Geometry check sheet. Reference: drawing and pictorial views, mm from the part's lowest x, y, z. A direction names the side the tool comes from. Give positions to 0.01 mm unless a question says otherwise; leave off trailing zeros. Write each loop counter-clockwise with the first axis right and the second up, starting at its lowest first coordinate (ties: lowest second). Pieces come first, ordered by that corner, then holes. Notation, with made-up numbers: (84, 12.5) -> (113, 12.5) arc R25 ccw to (113, 31.5) -> close; hole circle Ø9 at (2.5, 57.25). An arc over 180 degrees is marked (long way). Answer as CSV lines item,"result".
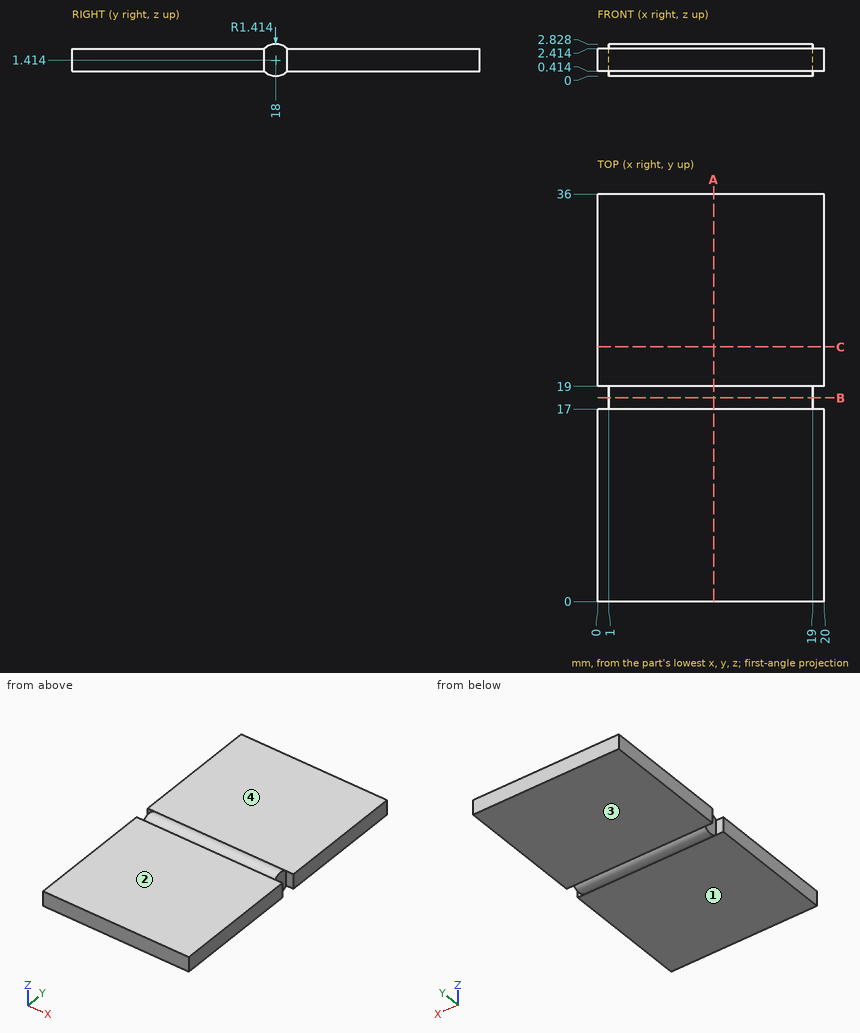
1) Section check B-B (y = 18). Record the boundary of the cut face in (x, z), and give its area (3 significant figures).
Reported:
outline,"(1, 0) -> (19, 0) -> (19, 2.83) -> (1, 2.83) -> close"
area,"50.9 mm²"
2) Section check C-C (y = 22.5). Record the boundary of the cut face in (x, z) (1 decimal), and give its area (3 significant figures).
Reported:
outline,"(0, 0.4) -> (20, 0.4) -> (20, 2.4) -> (0, 2.4) -> close"
area,"40.0 mm²"
3) Scan lines: line 1 along Z through (x, y) = (6.5, 12.5) (1 decimal); line 2 along Y through (x, z) = (6.75, 2.65) (1 decimal); line 3 along Y through (x, z) = (16, 2.5) (1 decimal). Record each from-to range of solid material in increasing order.
Reported:
line 1,"0.4 to 2.4"
line 2,"17.3 to 18.7"
line 3,"17.1 to 18.9"
4) Tool access check on the marked faces 1, 2, 3 and 4. Record the directions out of +Z, -Z, +X, -X, +Y, -Y that give a thin tool (end or side, any length) a straight path to the whole face; none if there is none.
Reported:
face 1,"-Z, +X, -X, -Y"
face 2,"+Z, +X, -X, -Y"
face 3,"-Z, +X, -X, +Y"
face 4,"+Z, +X, -X, +Y"
5) Depth check by flat-ended pin: pin 1 (1.6 mm diameter, centred on y = 18, z = 1, fed in from -X); pin 2 (1.5 mm diameter, centred on x = 2, y = 24.5, fed in from +Z); pin 3 (5 mm diameter, centred on x = 6.5, y = 7.5, fed in from -Z). Enter the tip coordinate at first touch or a pass-through.
Reported:
pin 1,"x = 1"
pin 2,"z = 2.41"
pin 3,"z = 0.41"
6) Section check A-A (x = 10.25). Record the boundary of the cut face in (y, z) (1 decimal).
Reported:
outline,"(0, 0.4) -> (17, 0.4) arc R1.4 ccw to (19, 0.4) -> (36, 0.4) -> (36, 2.4) -> (19, 2.4) arc R1.4 ccw to (17, 2.4) -> (0, 2.4) -> close"
